```python
from build123d import *

# Parameters (mm, degrees)
F0_W     = 22
F0_H     = 25
F1_DEPTH = 12
F2_W     = 17.8
F2_H     = 22
F3_DEPTH = 6
F5_DEPTH = 6
F6_R     = 1.6
F7_DEPTH = 6.001
F9_DEPTH = 3.5


with BuildPart() as f1:
    # F0 (on Front) → F1 (new body)
    with BuildSketch(Plane.XZ):
        with Locations((0, 12.5)):
            Rectangle(F0_W, F0_H)
    extrude(amount=-F1_DEPTH)

    # F2 (on face) → F3 (cut)
    with BuildSketch(Plane.XZ):
        with Locations((0, 14)):
            Rectangle(F2_W, F2_H)
    extrude(amount=-F3_DEPTH, mode=Mode.SUBTRACT)

    # F4 (on face) → F5 (join, through all)
    with BuildSketch(Plane.XZ):
        Polygon((-5.9, 14), (-8.9, 14), (-8.9, 9.3), (-5.9, 12.3), align=None)
        Polygon((8.9, 9.3), (8.9, 25), (5.9, 22), (5.9, 12.3), align=None)
    extrude(amount=-F5_DEPTH)

    # F6 (on face) → F7 (cut, through all)
    with BuildSketch(Plane.XZ.offset(-6)):
        with Locations((-1.7, 20.35)):
            Circle(F6_R)
    extrude(amount=-F7_DEPTH, mode=Mode.SUBTRACT)

    # F8 (on face) → F9 (cut)
    with BuildSketch(Plane(origin=(0, 12, 0), x_dir=(-1, 0, 0), z_dir=(0, 1, 0))):
        Polygon((4.65, 18.646817), (4.65, 22.053183), (1.7, 23.756367), (-1.25, 22.053183), (-1.25, 18.646817), (1.7, 16.943633), align=None)
    extrude(amount=-F9_DEPTH, mode=Mode.SUBTRACT)


solid = f1.part
```
Design review of the part built by this model. Coordinates are the model's own, in mm. A direction names the side the tool comes from. Round coordinates to 2 decimals unless told otherwise and drop trailing zeros. Write each loop counter-clockwise with the first axis right and the second up, starting at its lowest first coordinate (ties: lowest second). Pieces come first, ordered by that corner, then holes.
Item 1: We need section C-C on x = -1.25. Write out the cut boundary in (y, z).
Item 2: We need section B-B on x = -7.25. Write out the cut boundary in (y, z), and give its area (3 significant figures).
Item 3: Clearance check with flat-ended pins moving along their axes: pin 1 Ø3 at (x, z) = (1, 11.5) entering from -Y; pin 2 Ø1.9 at (x, z) = (-1.7, 20.35) entering from -Y; pin 3 Ø1.8 at (x, y) = (-1.5, 3.5) entering from +Z. State where each tip first meets the part, or that it passes through.
Item 4: We need section A-A on z = 20.35. Write out the cut boundary in (x, y), and give its area (3 significant figures).
Item 5: We need section D-D on y = 2. Write out the cut boundary in (x, z), and give its area (3 significant figures).
Item 6: The part is to be moulded in two halves that separate along Z. For faces 1 (the flat face through (0, 9, 25)), 2 (the flat face through (0, 12, 13)), 3 (the flat face through (0, 8.5, 19)), say which applies: +Z half, -Z half, draft (parallel to the pull), parting line (faces both ways), or undercut.
Item 7: For probe 1 along Z at (x, y) = (-1.7, 7.5); probe 2 along X at (y, z) = (2.75, 18); probe 3 along Y at (x, z) = (2.25, 15.5), list the stretches that pass through material, from the lowest coordinate up.
Item 8: For faces 4 (the flat face through (7.4, 3, 23.5)), 5 (the flat face through (-0.25, 10.27, 22.92)), 6 (the flat face through (0, 3, 3)), list the 3-axis set-ups (+Z, -Z, +X, -X, +Y, -Y) from which the entire face can be reached by the end or side of a thin tool; tool diameter is ignored.
Returned:
1. outline: (0, 0) - (12, 0) - (12, 17.2) - (8.5, 17.2) - (8.5, 18.81) - (6, 18.81) - (6, 3) - (0, 3) - close; (6, 21.89) - (8.5, 21.89) - (8.5, 23.5) - (12, 23.5) - (12, 25) - (6, 25) - close
2. outline: (0, 0) - (12, 0) - (12, 25) - (6, 25) - (6, 14) - (0, 14) - (0, 10.95) - (6, 10.95) - (6, 3) - (0, 3) - close
2. area: 186 mm2
3. pin 1: stops at y = 6
3. pin 2: passes through
3. pin 3: stops at z = 3
4. outline: (-11, 0) - (-8.9, 0) - (-8.9, 6) - (-3.3, 6) - (-3.3, 8.5) - (-4.65, 8.5) - (-4.65, 12) - (-11, 12) - close; (-0.1, 6) - (5.9, 6) - (5.9, 0) - (11, 0) - (11, 12) - (1.25, 12) - (1.25, 8.5) - (-0.1, 8.5) - close
4. area: 147 mm2
5. outline: (-11, 0) - (11, 0) - (11, 25) - (8.9, 25) - (5.9, 22) - (5.9, 12.3) - (8.9, 9.3) - (8.9, 3) - (-8.9, 3) - (-8.9, 9.3) - (-5.9, 12.3) - (-5.9, 14) - (-8.9, 14) - (-8.9, 25) - (-11, 25) - close
5. area: 206 mm2
6. face 1: +Z half
6. face 2: draft
6. face 3: undercut
7. probe 1: z = 0 to 18.75, 21.95 to 25
7. probe 2: x = -11 to -8.9, 5.9 to 11
7. probe 3: y = 6 to 12
8. face 4: +Z, -Y
8. face 5: +Y
8. face 6: -Y
